Source: CAD feature listing. Evaluate the final solid. Frame: model axes, mm. Give positions to 0.01 mm unless a question says otherwise; leave off trailing zeros. Order: outer loops, then holes, each group sorted by start corner. A loop starts at its lowest first (then second) coordinate and runs counter-clockwise, first axis right, second up. Notation, with made-up numbers: (-38, 79.5) -> (-29, 79.5) arc R22 ccw to (-29, 97.5) -> close; hole circle Ø10 at (39.25, 27.5). An arc over 180 degrees is marked (long way). Answer in a Markdown table with one row per item.
```python
from build123d import *

# Parameters (mm, degrees)
F0_R     = 5.715
F1_DEPTH = 8.89


# Not quite as in the source:
# - the program builds the solid bodies; features that only make, move or delete a surface that nothing else refers to are left out


with BuildPart() as f1:
    # F0 (on Top) → F1 (new body)
    with BuildSketch(Plane.XY):
        with BuildLine():
            ThreePointArc((-87.9825091655, 10.033), (-80.8881068298, 7.0944023356), (-77.9495091655, 0))
            ThreePointArc((-77.9495091655, 0), (-80.8881068298, -7.0944023356), (-87.9825091655, -10.033))
            Line((-87.9825091655, -10.033), (26.3174908345, -10.033))
            ThreePointArc((26.3174908345, -10.033), (16.2844908345, 0), (26.3174908345, 10.033))
            Line((26.3174908345, 10.033), (-87.9825091655, 10.033))
        make_face()
        with BuildLine():
            ThreePointArc((-87.9825091655, -10.033), (-80.8881068298, -7.0944023356), (-77.9495091655, 0))
            ThreePointArc((-77.9495091655, 0), (-80.8881068298, 7.0944023356), (-87.9825091655, 10.033))
            ThreePointArc((-87.9825091655, 10.033), (-98.0155091655, 0), (-87.9825091655, -10.033))
        make_face()
        with Locations((-87.9825091655, 0)):
            Circle(F0_R, mode=Mode.SUBTRACT)
        with BuildLine():
            ThreePointArc((36.3504908345, 0), (33.4118931702, 7.0944023356), (26.3174908345, 10.033))
            ThreePointArc((26.3174908345, 10.033), (16.2844908345, 0), (26.3174908345, -10.033))
            ThreePointArc((26.3174908345, -10.033), (33.4118931702, -7.0944023356), (36.3504908345, 0))
        make_face()
        with Locations((26.3174908345, 0)):
            Circle(F0_R, mode=Mode.SUBTRACT)
    extrude(amount=F1_DEPTH)


solid = f1.part
```
(1) Ray query, probe 1 along X at (y, z) = (-3.5, 1); probe 2 along X at (y, z) = (-4.25, 4); probe 3 along Y at (x, z) = (-83, 3.25). Return the intervals inside material, ascending.
A:
| item | result |
|---|---|
| probe 1 | x = -97.39 to -92.5, -83.46 to 21.8, 30.84 to 35.72 |
| probe 2 | x = -97.07 to -91.8, -84.16 to 22.5, 30.14 to 35.41 |
| probe 3 | y = -10.03 to -2.8, 2.8 to 10.03 |
(2) Section query B-B (y = 2.5). Return the cut outline in (x, z).
A:
| item | result |
|---|---|
| outline | (-97.7, 0) -> (-93.12, 0) -> (-93.12, 8.89) -> (-97.7, 8.89) -> close; (-82.84, 0) -> (21.18, 0) -> (21.18, 8.89) -> (-82.84, 8.89) -> close; (31.46, 0) -> (36.03, 0) -> (36.03, 8.89) -> (31.46, 8.89) -> close |
(3) First-contact query: pin 1 Ø9 at (x, y) = (-87.98, 0) entering from -Z; pin 2 Ø6 at (x, y) = (-65.5, 0.5) entering from -Z; pin 3 Ø5 at (y, z) = (-7.5, 6.5) entering from -X; pin 4 Ø1.5 at (y, z) = (-2, 5.5) entering from +X. Flat tips, straight axial feed; report the tip coordinate or a pass-through.
A:
| item | result |
|---|---|
| pin 1 | passes through |
| pin 2 | stops at z = 0 |
| pin 3 | stops at x = -96.68 |
| pin 4 | stops at x = 36.27 |
(4) Section query A-A (z = 1.5). Return the cut outline in (x, y) (1 decimal), plus the area to 3 significant figures.
A:
| item | result |
|---|---|
| outline | (-88, -10) -> (26.3, -10) arc R10 ccw to (26.3, 10) -> (-88, 10) arc R10 ccw to start; hole circle Ø11.4 at (-88, 0); hole circle Ø11.4 at (26.3, 0) |
| area | 2,400 mm^2 |
(5) Section query C-C (y = 8). Return the cut outline in (x, z), plus the area to 3 significant figures.
A:
| item | result |
|---|---|
| outline | (-94.04, 0) -> (32.37, 0) -> (32.37, 8.89) -> (-94.04, 8.89) -> close |
| area | 1,120 mm^2 |
(6) Pull-direction query (X, two-part tool) for faces 1 (the flat face through (-32, 0, 0)), 2 (the cylindrical face through (-98.013, 0.221, 4.383)), 3 (the cylindrical face through (29.39, 4.82, 4.38)); classes: +X half, -X half, draft (parallel to the pull), parting line (faces both ways), or undercut.
A:
| item | result |
|---|---|
| face 1 | draft |
| face 2 | -X half |
| face 3 | undercut |
